Source: CAD feature listing. Evaluate the final solid. Frame: model axes, mm. Face numbers are marked on the shaded views. A direction names the side the tool comes from. Round coordinates to 2 decimals unless told otherwise and drop trailing zeros. Order: outer loops, then holes, each group sorted by start corner. A loop starts at its lowest first (then second) coordinate and runs counter-clockwise, first axis right, second up. Notation, with made-up numbers: (89.5, 59.25) - (113.5, 59.25) arc R36 cw to (113.5, 98.25) - close; hole circle Ø5 at (-21.5, 15). An arc over 180 degrees is marked (long way). Return JSON: item names as keys, results as strings. Group by question number.
1) Mould query, pull axis Y, two halves, no side actions, for the marked faces 1, 2, 3 and 4. Classes: pulls with the +Y half, pulls with the -Y half, needs draft (parallel to the pull), parting line crosses it, or undercut.
2) Section C-C, the plane x = 20. Return loops of the section in (y, z).
3) Contact query for flat-ended pins moving along their axis: P1, Ø1.5, axis at x = 18, y = 8, coming from the -Z side; P2, Ø1.2, axis at y = 9.5, z = -26, coming from the +X side; P3, Ø4, axis at y = 5.5, z = -3.5, coming from the -X side; P4, Ø2.5, axis at x = 20, z = -15, coming from the -Y side. Output: stop coordinate, or through.
4) Ray query, line 1 (Z direction, x = 20, y = 8); line 2 (X direction, y = 8.25, z = 15); line 3 (Z direction, x = -13.5, y = 10.75). Return the intervals inside material, ascending. Write a range as from..to.
5) Section A-A, the plane y = 5.75. Return loops of the section in (x, z), plus the area to 3 significant figures.
6) Section D-D, the plane z = -15. Return loops of the section in (x, y), plus the area to 3 significant figures.
7) Section B-B, the plane z = 11. Return loops of the section in (x, y).
8) Access query for the marked faces 5 and 6. Directions: +Z, -Z, +X, -X, +Y, -Y. A direction counts if a zero-diameter tool reaches every point of the face in a straight line with its end or side. Return the directions, or none.
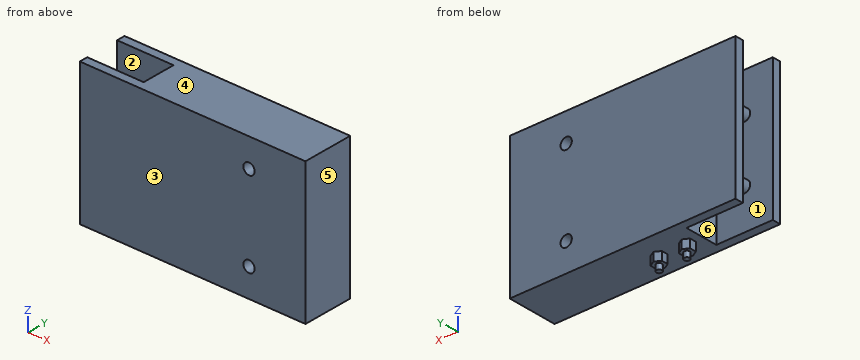
```python
from build123d import *

# Parameters (mm, degrees)
SKETCH1_W           = 80
SKETCH1_H           = 50
BOSS_EXTRUDE1_DEPTH = 3
SKETCH2_R           = 2
BOSS_EXTRUDE2_DEPTH = 14
SKETCH3_W           = 60
SKETCH3_H           = 50
BOSS_EXTRUDE3_DEPTH = 12
SKETCH4_R           = 3
CUT_EXTRUDE1_DEPTH  = 10
SKETCH5_W           = 80
SKETCH5_H           = 50
BOSS_EXTRUDE4_DEPTH = 3
SKETCH6_R           = 2
CUT_EXTRUDE2_DEPTH  = 49
BOSS_EXTRUDE5_DEPTH = 3
SKETCH8_R           = 1
BOSS_EXTRUDE6_DEPTH = 2


with BuildPart() as part:
    # Sketch1 → Boss-Extrude1 (new body)
    with BuildSketch(Plane(origin=(0, 0, 0), x_dir=(1, 0, 0), z_dir=(0, 1, 0))):
        Rectangle(SKETCH1_W, SKETCH1_H)
    extrude(amount=BOSS_EXTRUDE1_DEPTH)

    # Sketch2 → Boss-Extrude2 (add)
    with BuildSketch(Plane(origin=(0, 3, 0), x_dir=(1, 0, 0), z_dir=(0, 1, 0))):
        with Locations((-30, 11)):
            Circle(SKETCH2_R)
        with Locations((-30, -11)):
            Circle(SKETCH2_R)
    extrude(amount=BOSS_EXTRUDE2_DEPTH)

    # Sketch3 → Boss-Extrude3 (add)
    with BuildSketch(Plane(origin=(0, 3, 0), x_dir=(1, 0, 0), z_dir=(0, 1, 0))):
        with Locations((10, 0)):
            Rectangle(SKETCH3_W, SKETCH3_H)
    extrude(amount=BOSS_EXTRUDE3_DEPTH)

    # Sketch4 → Cut-Extrude1 (cut)
    with BuildSketch(Plane.ZY.offset(20)):
        with Locations((0, 11)):
            Circle(SKETCH4_R)
    extrude(amount=-CUT_EXTRUDE1_DEPTH, mode=Mode.SUBTRACT)

    # Sketch5 → Boss-Extrude4 (add)
    with BuildSketch(Plane(origin=(0, 15, 0), x_dir=(1, 0, 0), z_dir=(0, 1, 0))):
        Rectangle(SKETCH5_W, SKETCH5_H)
    extrude(amount=BOSS_EXTRUDE4_DEPTH)

    # Sketch6 → Cut-Extrude2 (cut)
    with BuildSketch(Plane(origin=(0, 18, 0), x_dir=(1, 0, 0), z_dir=(0, 1, 0))):
        with Locations((20, 15)):
            Circle(SKETCH6_R)
        with Locations((20, -15)):
            Circle(SKETCH6_R)
    extrude(amount=-CUT_EXTRUDE2_DEPTH, mode=Mode.SUBTRACT)

    # Sketch7 → Boss-Extrude5 (add)
    with BuildSketch(Plane(origin=(0, 0, -25), x_dir=(-1, 0, 0), z_dir=(0, 0, -1))):
        Polygon((15, 11.309401077), (13, 10.154700538), (13, 7.845299462), (15, 6.690598923), (17, 7.845299462), (17, 10.154700538), align=None)
        Polygon((5, 11.309401077), (3, 10.154700538), (3, 7.845299462), (5, 6.690598923), (7, 7.845299462), (7, 10.154700538), align=None)
    extrude(amount=BOSS_EXTRUDE5_DEPTH)

    # Sketch8 → Boss-Extrude6 (add)
    with BuildSketch(Plane(origin=(0, 0, -28), x_dir=(-1, 0, 0), z_dir=(0, 0, -1))):
        with Locations((14.883913009, 9)):
            Circle(SKETCH8_R)
        with Locations((5, 9)):
            Circle(SKETCH8_R)
    extrude(amount=BOSS_EXTRUDE6_DEPTH)


solid = part.part
```
Geometry check:
{
 "1": {"face 1": "undercut", "face 2": "undercut", "face 3": "pulls with the -Y half", "face 4": "needs draft"},
 "2": {"outline": "(0, -25) - (18, -25) - (18, -17) - (0, -17) - close; (0, -13) - (18, -13) - (18, 13) - (0, 13) - close; (0, 17) - (18, 17) - (18, 25) - (0, 25) - close"},
 "3": {"P1": "z = -25", "P2": "x = -3", "P3": "x = -20", "P4": "through"},
 "4": {"line 1": "-25..-17, -13..13, 17..25", "line 2": "-20..18, 22..40", "line 3": "-25..-2.99, 2.99..25"},
 "5": {"outline": "circle Ø4 at (-30, -11); circle Ø4 at (-30, 11); (-20, -25) - (40, -25) - (40, 25) - (-20, 25) - close; hole circle Ø4 at (20, -15); hole circle Ø4 at (20, 15)", "area": "3,000 mm2"},
 "6": {"outline": "(-40, 0) - (18, 0) - (18, 18) - (-40, 18) - (-40, 15) - (-20, 15) - (-20, 3) - (-40, 3) - close; (22, 0) - (40, 0) - (40, 18) - (22, 18) - close", "area": "1,130 mm2"},
 "7": {"outline": "(-40, 0) - (40, 0) - (40, 18) - (-40, 18) - (-40, 15) - (-32, 15) - (-32, 3) - (-40, 3) - close; hole (-28, 3) - (-20, 3) - (-20, 15) - (-28, 15) - close"},
 "8": {"face 5": "+Z, -Z, +X, +Y, -Y", "face 6": "+Z, -Z"}
}
